Job drawing, mm, ordinate dimensions from the low corner. One solid piece. Round coordinates to 2 decimals unless told otherwise and drop trailing zeros. Loops run counter-clockwise (first coordinate to the right, second up) from the corner with the lowest first, then second, coordinate; pieces in that order, holes last.
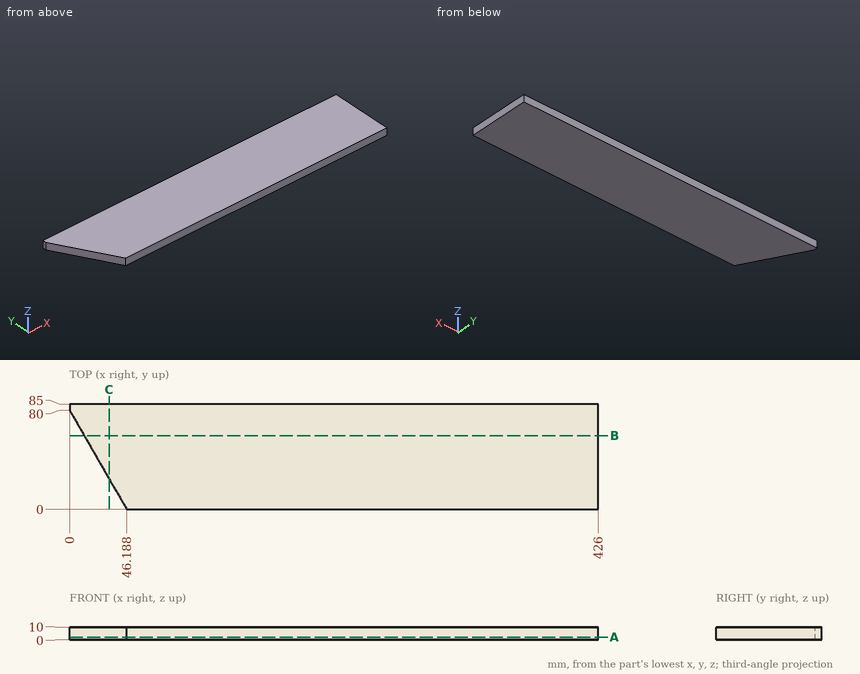
1) Wall check: line 1 along X through (y, z) = (41, 6); line 2 along X through (y, z) = (67.5, 2); line 3 along Y through (x, z) = (38, 3.5). Give the ranges that are in metal, low to high.
Values:
line 1: x = 22.52 to 426
line 2: x = 7.22 to 426
line 3: y = 14.18 to 85
2) Slice it at C-C, the plane x = 32. Give the cut face in (y, z), then the cut area to 3 significant figures.
Values:
outline: (24.57, 0) - (85, 0) - (85, 10) - (24.57, 10) - close
area: 604 mm2
3) Slice it at B-B, the plane y = 59.5. Give the cut face in (x, z), then the cut area to 3 significant figures.
Values:
outline: (11.84, 0) - (426, 0) - (426, 10) - (11.84, 10) - close
area: 4,140 mm2
4) Slice it at A-A, the plane z = 2.25. Give the cut face in (x, y).
Values:
outline: (0, 80) - (46.19, 0) - (426, 0) - (426, 85) - (0, 85) - close
5) Drop flat-ended pins along their axis: pin 1 Ø6 at (x, y) = (202.5, 71.5) entering from -Z; pin 2 Ø2 at (y, z) = (41, 5.5) entering from -X. Give the stop position or say it passes through.
Values:
pin 1: stops at z = 0
pin 2: stops at x = 21.94
